from build123d import *

# Parameters (mm, degrees)
ESQUISSE1_R             = 7
ESQUISSE1_R_2           = 1.8
BOSS_EXTRU_1_DEPTH      = 8
ESQUISSE2_R             = 13.4
ENL_V_MAT_EXTRU_1_DEPTH = 6
ESQUISSE3_R             = 2
ENL_V_MAT_EXTRU_2_DEPTH = 12
CHANFREIN1_SIZE         = 1


with BuildPart() as part:
    # Esquisse1 → Boss.-Extru.1 (new body)
    with BuildSketch(Plane.XY):
        with BuildLine():
            Line((-20, 0), (-20, -25))
            Line((-20, -25), (20, -25))
            Line((20, -25), (20, 0))
            ThreePointArc((20, 0), (0, 20), (-20, 0))
        make_face()
        Circle(ESQUISSE1_R, mode=Mode.SUBTRACT)
        with Locations((0, 10)):
            Circle(ESQUISSE1_R_2, mode=Mode.SUBTRACT)
        with Locations((10, 0)):
            Circle(ESQUISSE1_R_2, mode=Mode.SUBTRACT)
        with Locations((0, -10)):
            Circle(ESQUISSE1_R_2, mode=Mode.SUBTRACT)
        with Locations((-10, 0)):
            Circle(ESQUISSE1_R_2, mode=Mode.SUBTRACT)
    extrude(amount=BOSS_EXTRU_1_DEPTH)

    # Esquisse2 → Enlèv. mat.-Extru.1 (cut)
    with BuildSketch(Plane.XY.offset(8)):
        Circle(ESQUISSE2_R)
    extrude(amount=-ENL_V_MAT_EXTRU_1_DEPTH, mode=Mode.SUBTRACT)

    # Esquisse3 → Enlèv. mat.-Extru.2 (cut)
    with BuildSketch(Plane.XZ.offset(25)):
        with Locations((-15, 4)):
            Circle(ESQUISSE3_R)
        with Locations((15, 4)):
            Circle(ESQUISSE3_R)
    extrude(amount=-ENL_V_MAT_EXTRU_2_DEPTH, mode=Mode.SUBTRACT)

    # Chanfrein1
    chanfrein1_edges = [part.edges().sort_by_distance(p)[0] for p in [
        (-17, -25, 4),
        (13, -25, 4),
    ]]
    chamfer(chanfrein1_edges, length=CHANFREIN1_SIZE)


solid = part.part
Could you check a few things on this model? Use its own coordinates, in mm. A direction names the side the tool comes from. Coordinates: 2 decimals unless noted, no trailing zeros. Order: outer loops, then holes, each group sorted by start corner. A loop starts at its lowest first (then second) coordinate and runs counter-clockwise, first axis right, second up. Notation, with made-up numbers: (46, 16.25) - (98, 16.25) arc R20 cw to (98, 23.25) - close; hole circle Ø2 at (20, 56.25). An arc over 180 degrees is marked (long way). Answer in a Markdown table with one row per item. Add a question column.
(1) I need wall thicknesses on L1, parallel to Y at x = 0, z = 1.05; L2, parallel to X at y = -10, z = 1.1; L3, parallel to Y at x = 0, z = 3.75. Which ranges of each line are inside material? Lowest first, please.
(2) If we section it at A-A, the plane x = 0: Please give me the cut outline in (y, z), then the cut area to 3 significant figures.
(3) Will these pins go through, and if not, where does the flat tip stop? pin 1 (6 mm diameter, centred on x = -10, y = 0, fed in from +Z); pin 2 (4 mm diameter, centred on x = 6.5, z = 4.5, fed in from +Y); pin 3 (1.2 mm diameter, centred on x = 15, z = 5, fed in from -Y).
(4) On a 3-axis mill with a long thin cutter (end or side, diameter ignored), from which of +Z, -Z, +X, -X, +Y, -Y can I reach the whole of each face in a straight line? I mean faces 5 (the face through (-15, -13, 4)), 6 (the face through (6, -6, 2)), 7 (the face through (8.2, 0.08, 0.99)). Say none if no direction works.
(5) If we section it at B-B, the plane y = -14: Please give me the cut outline in (x, z), then the cut area to 3 significant figures.
(6) If we section it at C-C, the plane y = 6: Please give me the cut outline in (x, z).
(7) If we mould it in two halves opening along X, with no side actions, what happens to faces 1 (the face through (-15, -19, 2)), 2 (the face through (-0.3, -7.2, 0)), 3 (the face through (-0.39, -11.757, 0.986)), 4 (the face through (20, -13, 4))? For each: released by +X, released by -X, zero draft, split by the parting line, or undercut.
(8) If we section it at D-D, the plane x = -10: Please give me the cut outline in (y, z).
Results are:
| question | item | result |
|---|---|---|
| 1 | L1 | y = -25 to -11.8, -8.2 to -7, 7 to 8.2, 11.8 to 20 |
| 1 | L2 | x = -20 to -1.8, 1.8 to 20 |
| 1 | L3 | y = -25 to -13.4, 13.4 to 20 |
| 2 | outline | (-25, 0) - (-11.8, 0) - (-11.8, 2) - (-13.4, 2) - (-13.4, 8) - (-25, 8) - close; (-8.2, 0) - (-7, 0) - (-7, 2) - (-8.2, 2) - close; (7, 0) - (8.2, 0) - (8.2, 2) - (7, 2) - close; (11.8, 0) - (20, 0) - (20, 8) - (13.4, 8) - (13.4, 2) - (11.8, 2) - close |
| 2 | area | 157 mm2 |
| 3 | pin 1 | stops at z = 2 |
| 3 | pin 2 | stops at y = 19.49 |
| 3 | pin 3 | stops at y = -13 |
| 4 | face 5 | -Y |
| 4 | face 6 | +Z |
| 4 | face 7 | +Z, -Z |
| 5 | outline | (-20, 0) - (20, 0) - (20, 8) - (-20, 8) - close; hole circle Ø4 at (-15, 4); hole circle Ø4 at (15, 4) |
| 5 | area | 295 mm2 |
| 6 | outline | (-19.08, 0) - (-3.61, 0) - (-3.61, 2) - (-11.98, 2) - (-11.98, 8) - (-19.08, 8) - close; (3.61, 0) - (19.08, 0) - (19.08, 8) - (11.98, 8) - (11.98, 2) - (3.61, 2) - close |
| 7 | face 1 | undercut |
| 7 | face 2 | zero draft |
| 7 | face 3 | undercut |
| 7 | face 4 | released by +X |
| 8 | outline | (-25, 0) - (-1.8, 0) - (-1.8, 2) - (-8.92, 2) - (-8.92, 8) - (-25, 8) - close; (1.8, 0) - (17.32, 0) - (17.32, 8) - (8.92, 8) - (8.92, 2) - (1.8, 2) - close |
